```python
from build123d import *

# Parameters (mm, degrees)
CROQUIS1_W              = 70
CROQUIS1_H              = 130
SALIENTE_EXTRUIR1_DEPTH = 5
REDONDEO1_R             = 10
CROQUIS2_R              = 5
SALIENTE_EXTRUIR3_DEPTH = 23
CROQUIS3_W              = 30
CROQUIS3_H              = 5
SALIENTE_EXTRUIR4_DEPTH = 30
CROQUIS5_R              = 10
CORTAR_EXTRUIR2_DEPTH   = 112.579568022
REDONDEO2_R             = 10
REDONDEO3_R             = 10


with BuildPart() as part:
    # Croquis1 → Saliente-Extruir1 (new, symmetric)
    with BuildSketch(Plane.XY):
        Rectangle(CROQUIS1_W, CROQUIS1_H)
    extrude(amount=SALIENTE_EXTRUIR1_DEPTH, both=True)

    # Redondeo1
    redondeo1_edges = [part.edges().sort_by_distance(p)[0] for p in [
        (35, -65, 0),
        (-35, -65, 0),
        (-35, 65, 0),
        (35, 65, 0),
    ]]
    fillet(redondeo1_edges, radius=REDONDEO1_R)

    # Croquis2 → Saliente-Extruir3 (add)
    with BuildSketch(Plane.XY.offset(5)):
        with Locations((0, -25)):
            Circle(CROQUIS2_R)
    extrude(amount=SALIENTE_EXTRUIR3_DEPTH)

    # Croquis3 → Saliente-Extruir4 (add)
    with BuildSketch(Plane.XY.offset(35)):
        with Locations((0, 62.5)):
            Rectangle(CROQUIS3_W, CROQUIS3_H)
        with Locations((0, 37.5)):
            Rectangle(CROQUIS3_W, CROQUIS3_H)
    extrude(amount=-SALIENTE_EXTRUIR4_DEPTH)

    # Croquis5 → Cortar-Extruir2 (cut, through all)
    with BuildSketch(Plane.XZ.offset(-35)):
        with Locations(Location((0, 20, 0), (0, 0, 270))):
            Circle(CROQUIS5_R)
    extrude(amount=-CORTAR_EXTRUIR2_DEPTH, mode=Mode.SUBTRACT)

    # Redondeo2
    redondeo2_edges = [part.edges().sort_by_distance(p)[0] for p in [
        (-15, 62.5, 5),
        (-15, 62.5, 35),
        (15, 62.5, 5),
        (15, 62.5, 35),
    ]]
    fillet(redondeo2_edges, radius=REDONDEO2_R)

    # Redondeo3
    redondeo3_edges = [part.edges().sort_by_distance(p)[0] for p in [
        (-15, 37.5, 5),
        (15, 37.5, 5),
        (-15, 37.5, 35),
        (15, 37.5, 35),
    ]]
    fillet(redondeo3_edges, radius=REDONDEO3_R)


solid = part.part
```
Input: part model. Units: mm. Frame: model coordinates. A direction names the side the tool comes from. Round coordinates to 2 decimals unless told otherwise and drop trailing zeros. Loops run counter-clockwise (first coordinate to the right, second up) from the corner with the lowest first, then second, coordinate; pieces in that order, holes last. Notation, with made-up numbers: (34, 84.25) -> (78, 84.25) arc R25 cw to (78, 117.25) -> close; hole circle Ø5 at (66, 29). An arc over 180 degrees is marked (long way). One line per item, written item: value.
(1) Section D-D (x = -18). Return the cut outline in (y, z).
Geometry check:
outline: (-65, -5) -> (65, -5) -> (65, 7.86) -> (60, 7.86) -> (60, 5) -> (40, 5) -> (40, 7.86) -> (35, 7.86) -> (35, 5) -> (-65, 5) -> close
(2) Set-up query: faces 1 (the face through (15, 37, 20)), 2 (the face through (3, 62.46, 10.46)), 3 (the face through (-15, 62, 20)), 4 (the face through (-6, 60, 11)). Return all of +Z, -Z, +X, -X, +Y, -Y with unobstructed straight access to the full face (end or side cutting, diameter ignored); none if empty.
Geometry check:
face 1: +Z, +X, +Y, -Y
face 2: +Y
face 3: +Z, -X, +Y, -Y
face 4: +Z, +X, -X
(3) Section C-C (y = -25). Return the cut outline in (x, z).
Geometry check:
outline: (-35, -5) -> (35, -5) -> (35, 5) -> (5, 5) -> (5, 28) -> (-5, 28) -> (-5, 5) -> (-35, 5) -> close
(4) Pin query (flat end, axial travel): pin 1 (9 mm diameter, centred on x = -6, z = 16, fed in from -Y); pin 2 (16 mm diameter, centred on x = 0, z = 20, fed in from -Y); pin 3 (3 mm diameter, centred on x = 11, y = 37.5, fed in from +Z). Return the tip coordinate at first contact, or that it passes through.
Geometry check:
pin 1: y = -29.77
pin 2: y = -30
pin 3: z = 33.93
(5) Material intervals for line 1 (X direction, y = 62, z = 20); line 2 (Z direction, x = -29, y = 26); line 3 (Y direction, x = 10, z = 19), sorted ascending. Write a range as [from, to].
Geometry check:
line 1: [-15, -10], [10, 15]
line 2: [-5, 5]
line 3: [35, 40], [60, 65]
(6) Mould query, pull axis X, two halves, no side actions, for faces 5 (the face through (-1.08, -29.88, 16.34)), 6 (the face through (-35, -1, 0)), 7 (the face through (3, 37.47, 10.46)). Classes: pulls with the +X half, pulls with the -X half, needs draft (parallel to the pull), parting line crosses it, or undercut.
Geometry check:
face 5: parting line crosses it
face 6: pulls with the -X half
face 7: undercut
(7) Section B-B (z = 20). Return the cut outline in (x, y).
Geometry check:
outline: (-15, 35) -> (-10, 35) -> (-10, 40) -> (-15, 40) -> close; (-15, 60) -> (-10, 60) -> (-10, 65) -> (-15, 65) -> close; circle Ø10 at (0, -25); (10, 35) -> (15, 35) -> (15, 40) -> (10, 40) -> close; (10, 60) -> (15, 60) -> (15, 65) -> (10, 65) -> close
(8) Section A-A (x = 0). Return the cut outline in (y, z), plus the area to 3 significant figures.
Geometry check:
outline: (-65, -5) -> (65, -5) -> (65, 10) -> (60, 10) -> (60, 5) -> (40, 5) -> (40, 10) -> (35, 10) -> (35, 5) -> (-20, 5) -> (-20, 28) -> (-30, 28) -> (-30, 5) -> (-65, 5) -> close; (35, 30) -> (40, 30) -> (40, 35) -> (35, 35) -> close; (60, 30) -> (65, 30) -> (65, 35) -> (60, 35) -> close
area: 1,630 mm2
